```python
from build123d import *

# Parameters (mm, degrees)
BOSS_EXTRUDE1_DEPTH     = 30
CUT_EXTRUDE1_DEPTH      = 74.898579147
CUT_EXTRUDE1_DEPTH_BACK = 74.898579147
FILLET1_R               = 10
FILLET2_R               = 30
CUT_EXTRUDE2_DEPTH      = 73.01388755
CUT_EXTRUDE2_DEPTH_BACK = 73.01388755
FILLET3_R               = 10
SKETCH4_R               = 4
CUT_EXTRUDE3_DEPTH      = 90.827612681
FILLET4_R               = 4
SKETCH5_R               = 11
SKETCH5_R_2             = 7.5
CUT_EXTRUDE4_DEPTH      = 3
SKETCH5_2_R             = 7.5
CUT_EXTRUDE6_DEPTH      = 69.971008402


with BuildPart() as part:
    # Sketch1 → Boss-Extrude1 (new body)
    with BuildSketch(Plane.XY):
        with BuildLine():
            Line((-21, 48.152987889), (-21, 60))
            Line((-21, 60), (-31, 60))
            Line((-31, 60), (-31, 48.152987889))
            ThreePointArc((-31, 48.152987889), (-30.537169507, 45.145929894), (-29.191520443, 42.417223525))
            Line((-29.191520443, 42.417223525), (-11.127260537, 16.618786747))
            ThreePointArc((-11.127260537, 16.618786747), (-13.173135996, 15.048869992), (-15, 13.228756555))
            Line((-15, 13.228756555), (-15, 0))
            Line((-15, 0), (15, 0))
            Line((15, 0), (15, 13.228756555))
            ThreePointArc((15, 13.228756555), (13.173135996, 15.048869992), (11.127260537, 16.618786747))
            Line((11.127260537, 16.618786747), (29.191520443, 42.417223525))
            ThreePointArc((29.191520443, 42.417223525), (30.537169507, 45.145929894), (31, 48.152987889))
            Line((31, 48.152987889), (31, 60))
            Line((31, 60), (21, 60))
            Line((21, 60), (21, 48.152987889))
            ThreePointArc((21, 48.152987889), (20.537169507, 45.145929894), (19.191520443, 42.417223525))
            Line((19.191520443, 42.417223525), (3.302564109, 19.725442208))
            ThreePointArc((3.302564109, 19.725442208), (0, 20), (-3.302564109, 19.725442208))
            Line((-3.302564109, 19.725442208), (-19.191520443, 42.417223525))
            ThreePointArc((-19.191520443, 42.417223525), (-20.537169507, 45.145929894), (-21, 48.152987889))
        make_face()
    extrude(amount=BOSS_EXTRUDE1_DEPTH)

    # Sketch2 → Cut-Extrude1 (cut, two sides: drawn at the far end of the back side and taken through both)
    with BuildSketch(Plane(origin=(0, 0, 0), x_dir=(0, 0, -1), z_dir=(1, 0, 0)).offset(-CUT_EXTRUDE1_DEPTH_BACK)):
        Polygon((-25, 0), (-25, 16.618786747), (-12, 42.417223525), (-12, 60), (-30, 60), (-30, 0), align=None)
    extrude(amount=CUT_EXTRUDE1_DEPTH + CUT_EXTRUDE1_DEPTH_BACK, mode=Mode.SUBTRACT)

    # Fillet1
    # the kernel refuses this fillet: 10 mm, written as the material it adds along each edge
    with BuildSketch(Plane(origin=(11.127260537, 16.618786747, 0), x_dir=(0.75244349959859, -0.6586567997916871, 0), z_dir=(0, 0, 1))) as fillet1_piece_1_section:
        with BuildLine():
            CenterArc((9.059445237, 9.202818325), FILLET1_R, 186.19751299, 60.769805767)
            Line((-0.882111272, 8.123256295), (-1.080942402, 8.101665055))
            Line((-1.080942402, 8.101665055), (-0.19883113, -0.021591241))
            Line((-0.19883113, -0.021591241), (0.02573442, -0.198337439))
            ThreePointArc((0.02573442, -0.198337439), (2.573442036, -0.033743875), (5.068632849, -0.184056367))
            Line((5.068632849, -0.184056367), (5.146884072, 0))
        make_face()
    fillet1_piece_1 = extrude(amount=25, mode=Mode.PRIVATE)
    fillet1_piece_1 = split(fillet1_piece_1, bisect_by=Plane(origin=(13.208648134, 22.312499117, 22.130901324), z_dir=(0, -0.4500023080786392, -0.8930273919224972)), keep=Keep.TOP, mode=Mode.PRIVATE)
    add(fillet1_piece_1)
    with BuildSketch(Plane(origin=(-11.127260537, 16.618786747, 0), x_dir=(-0.573576436351047, 0.819152044288991, 0), z_dir=(0, 0, 1))) as fillet1_piece_2_section:
        with BuildLine():
            CenterArc((8.171010533, 10), FILLET1_R, 209.230194233, 60.769805767)
            Line((-0.555638062, 5.116803885), (-0.730171033, 5.019139963))
            ThreePointArc((-0.730171033, 5.019139963), (-0.311365695, 2.554759082), (-0.199956476, 0.004172263))
            Line((-0.199956476, 0.004172263), (0, -0.2))
            Line((0, -0.2), (8.171010533, -0.2))
            Line((8.171010533, -0.2), (8.171010533, 0))
        make_face()
    fillet1_piece_2 = extrude(amount=25, mode=Mode.PRIVATE)
    fillet1_piece_2 = split(fillet1_piece_2, bisect_by=Plane(origin=(-15.334467923, 27.154175935, 19.691148901), z_dir=(0, -0.4500023080786392, -0.8930273919224972)), keep=Keep.TOP, mode=Mode.PRIVATE)
    add(fillet1_piece_2)

    # Fillet2
    fillet2_edges = [part.edges().sort_by_distance(p)[0] for p in [
        (-15, 13.228756555, 12.5),
        (15, 13.228756555, 12.5),
    ]]
    fillet(fillet2_edges, radius=FILLET2_R)

    # Sketch3 → Cut-Extrude2 (cut, two sides: drawn at the far end of the back side and taken through both)
    with BuildSketch(Plane(origin=(0, 0, 0), x_dir=(0, 0, -1), z_dir=(1, 0, 0)).offset(-CUT_EXTRUDE2_DEPTH_BACK)):
        Polygon((-14, 0), (-14, 15.360293774), (0, 42.417223525), (0, 0), align=None)
    extrude(amount=CUT_EXTRUDE2_DEPTH + CUT_EXTRUDE2_DEPTH_BACK, mode=Mode.SUBTRACT)

    # Fillet3
    # the kernel refuses this fillet: 10 mm, written as the material it adds along each edge
    with BuildSketch(Plane(origin=(3.302564109, 19.725442208, -1.95547457), x_dir=(-0.9985520834372477, 0.053793463014867454, 0), z_dir=(0, 0, 1))) as fillet3_piece_1_section:
        with BuildLine():
            CenterArc((5.591706065, -9.937268887), FILLET3_R, 96.421055445, 51.662571373)
            Line((-2.896500368, -4.650459684), (0, 0))
            ThreePointArc((0, 0), (2.236682426, -0.125462226), (4.473364852, 0))
        make_face()
    fillet3_piece_1 = extrude(amount=39.086837339, mode=Mode.PRIVATE)
    fillet3_piece_1 = split(fillet3_piece_1, bisect_by=Plane(origin=(3.109386203, 18.47326219, 12.38926448), z_dir=(0, 0.45955333907229245, 0.888150172294926)), keep=Keep.TOP, mode=Mode.PRIVATE)
    fillet3_piece_1 = split(fillet3_piece_1, bisect_by=Plane(origin=(3.109386203, 23.215327511, 21.675960227), z_dir=(0, -0.4500023080791268, -0.8930273919222517)), keep=Keep.TOP, mode=Mode.PRIVATE)
    add(fillet3_piece_1)
    with BuildSketch(Plane(origin=(-3.302564109, 19.725442208, -1.95547457), x_dir=(-0.5735764363510474, 0.8191520442889909, 0), z_dir=(0, 0, 1))) as fillet3_piece_2_section:
        with BuildLine():
            CenterArc((5.47873066, -10), FILLET3_R, 90, 51.662571373)
            ThreePointArc((-2.364982647, -3.797084431), (-1.075996396, -1.964871701), (0, 0))
            Line((0, 0), (5.47873066, 0))
        make_face()
    fillet3_piece_2 = extrude(amount=39.086837339, mode=Mode.PRIVATE)
    fillet3_piece_2 = split(fillet3_piece_2, bisect_by=Plane(origin=(-3.109386203, 18.47326219, 12.38926448), z_dir=(0, 0.45955333907229245, 0.888150172294926)), keep=Keep.TOP, mode=Mode.PRIVATE)
    fillet3_piece_2 = split(fillet3_piece_2, bisect_by=Plane(origin=(-3.109386203, 23.215327511, 21.675960227), z_dir=(0, -0.4500023080791268, -0.8930273919222517)), keep=Keep.TOP, mode=Mode.PRIVATE)
    add(fillet3_piece_2)

    # Sketch4 → Cut-Extrude3 (cut, through all)
    with BuildSketch(Plane(origin=(31, 0, 0), x_dir=(0, 0, -1), z_dir=(1, 0, 0))):
        with Locations((-6, 54.076493944)):
            Circle(SKETCH4_R)
    extrude(amount=-CUT_EXTRUDE3_DEPTH, mode=Mode.SUBTRACT)

    # Fillet4
    fillet4_edges = [part.edges().sort_by_distance(p)[0] for p in [
        (-26, 60, 0),
        (26, 60, 0),
        (26, 60, 12),
        (-26, 60, 12),
    ]]
    fillet(fillet4_edges, radius=FILLET4_R)

    # Mirror2: part across plane


with BuildPart() as part_1:
    add(part.part)
    add(part.part.mirror(Plane(origin=(0, 0, 30), x_dir=(0, 0, 1), z_dir=(0, 1, 0))))

    # Sketch5 → Cut-Extrude4 (cut)
    with BuildSketch(Plane(origin=(0, 0, 14), x_dir=(-1, 0, 0), z_dir=(0, 0, -1))):
        Circle(SKETCH5_R)
        Circle(SKETCH5_R_2, mode=Mode.SUBTRACT)
    extrude(amount=-CUT_EXTRUDE4_DEPTH, mode=Mode.SUBTRACT)

    # Sketch5<2> → Cut-Extrude6 (cut, through all)
    with BuildSketch(Plane(origin=(0, 0, 14), x_dir=(-1, 0, 0), z_dir=(0, 0, -1))):
        Circle(SKETCH5_2_R)
    extrude(amount=-CUT_EXTRUDE6_DEPTH, mode=Mode.SUBTRACT)


solid = part_1.part
```
The model under review builds one solid part; all positions refer to its coordinate system, in mm. A direction names the side the tool comes from. Coordinates: 2 decimals unless noted, no trailing zeros. Order: outer loops, then holes, each group sorted by start corner. A loop starts at its lowest first (then second) coordinate and runs counter-clockwise, first axis right, second up. Notation, with made-up numbers: (74.25, 7.25) -> (129.25, 7.25) arc R23 cw to (129.25, 23.25) -> close; hole circle Ø8 at (-29, -12). An arc over 180 degrees is marked (long way). Answer in a Markdown table with one row per item. Add a question column.
Item 1: Clearance check with flat-ended pins moving along their axes: pin 1 (4 mm diameter, centred on x = -1, z = 18, fed in from -Y); pin 2 (1 mm diameter, centred on x = -10, z = 21.5, fed in from -Y); pin 3 (1 mm diameter, centred on x = -3, y = -17, fed in from -Z). State where each tip first meets the part, or that it passes through.
Item 2: Machinability: for faces 4 (the cylindrical face through (30.524, 45.105, 5.916)), 5 (the flat face through (-22.596, 32.998, 10.662)), 6 (the flat face through (12.908, 33.443, 10.438)), which of the approach directions +Z, -Z, +X, -X, +Y, -Y give a long, thin tool a straight path to every point of the face, cutting with its end or side? Answer none if there is none.
Item 3: Mouldability with a two-part tool opening along Z and no side actions: class faces 1 (the cylindrical face through (-20.524, 45.105, 5.916)), 2 (the flat face through (-7.2, 2.6, 17)), 3 (the cylindrical face through (-25.93, 50.172, 6.867)) as +Z half, -Z half, draft (parallel to the pull), parting line (faces both ways), or undercut.
Item 4: We need section A-A on y = 0. Write out the cut boundary in (x, z).
Item 5: To check wall thickness, follow probe 1 along Y at (x, z) = (26.5, 6); probe 2 along Y at (x, z) = (-22.5, 9.5); probe 3 along Y at (x, z) = (-18, 18.25). State the ranges of each line that lie inside material, in increasing order.
Item 6: We need section C-C on z = 6. Give the number of separate pieces and of enclosed holes in the cut face, plus the area to 3 significant figures.
Item 7: We need section B-B on x = 9.5. Write out the cut boundary in (y, z), plus the area to 3 significant figures.
Item 8: We need section D-D on y = 21.5. Write out the cut boundary in (x, z).
Final values:
| question | item | result |
|---|---|---|
| 1 | pin 1 | stops at y = -21.15 |
| 1 | pin 2 | stops at y = -24.56 |
| 1 | pin 3 | stops at z = 12.89 |
| 2 | face 4 | +Z, -Z, +X |
| 2 | face 5 | +Z, -Z, -X |
| 2 | face 6 | +Z, -Z, +Y |
| 3 | face 1 | draft |
| 3 | face 2 | -Z half |
| 3 | face 3 | undercut |
| 4 | outline | (-15, 14) -> (-11, 14) -> (-11, 17) -> (-7.5, 17) -> (-7.5, 25) -> (-15, 25) -> close; (7.5, 17) -> (11, 17) -> (11, 14) -> (15, 14) -> (15, 25) -> (7.5, 25) -> close |
| 5 | probe 1 | y = -60 to -58.08, -50.08 to -38.57, 38.57 to 50.08, 58.08 to 60 |
| 5 | probe 2 | y = -59.71 to -56.01, -52.14 to -32.86, 32.86 to 52.14, 56.01 to 59.71 |
| 5 | probe 3 | y = -30.01 to -26.43, 26.43 to 30.01 |
| 6 | separate pieces | 8 |
| 6 | enclosed holes | 0 |
| 6 | area | 847 mm2 |
| 7 | outline | (-28.58, 7.16) -> (-15.36, 14) -> (-5.55, 14) -> (-5.55, 17) -> (5.55, 17) -> (5.55, 14) -> (15.36, 14) -> (28.58, 7.16) -> (28.58, 18.97) -> (16.62, 25) -> (-16.62, 25) -> (-28.58, 18.97) -> close |
| 7 | area | 614 mm2 |
| 8 | outline | (-14.81, 10.82) -> (-3.6, 10.82) -> (-3.6, 22.54) -> (-14.81, 22.54) -> close; (3.6, 10.82) -> (14.81, 10.82) -> (14.81, 22.54) -> (3.6, 22.54) -> close |
